Here's the drawing with two shaded views (mm, measured from the low corner). I have some questions. A direction names the side the tool comes from. Give positions to 0.01 mm unless a question says otherwise; leave off trailing zeros. Write each loop counter-clockwise with the first axis right and the second up, starting at its lowest first coordinate (ties: lowest second). Pieces come first, ordered by that corner, then holes. Notation, with made-up numbers: (58.25, -13.5) - (103.25, -13.5) arc R7 cw to (103.25, -3.5) - close; hole circle Ø2 at (19, 15.5). An arc over 180 degrees is marked (long way). Write item = value, one per line.
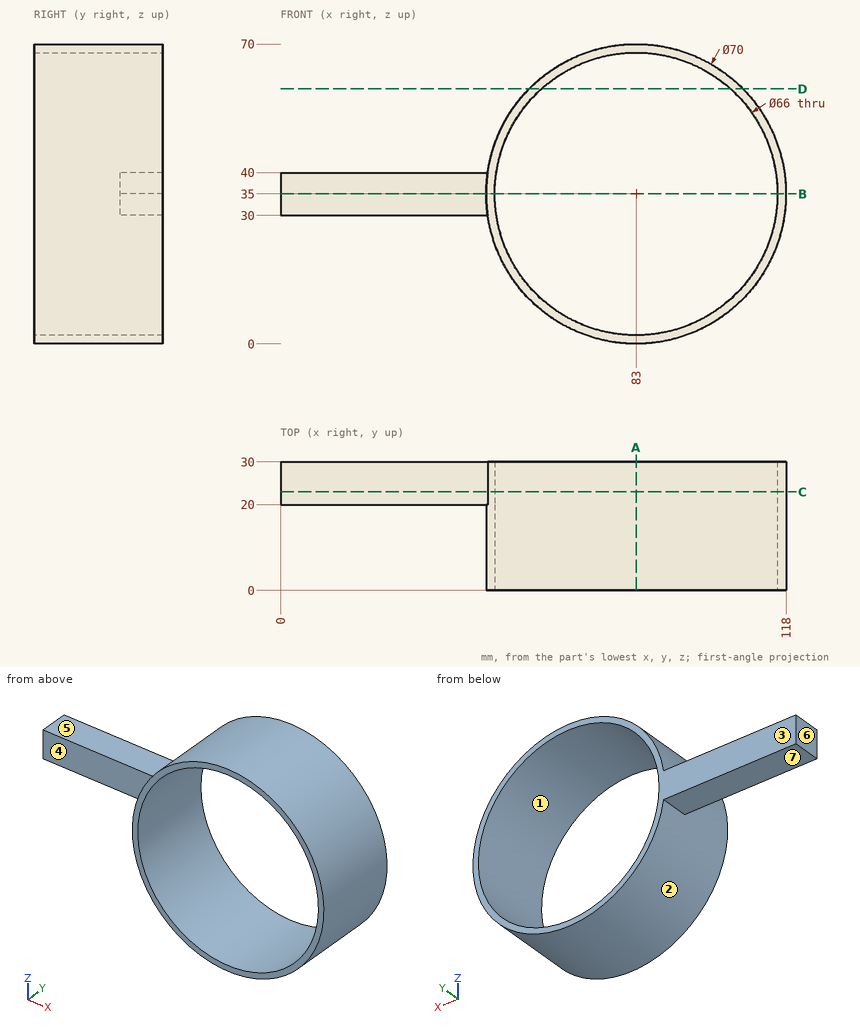
1. I need wall thicknesses on line 1 (Z direction, x = 83, y = 11.75); line 2 (X direction, y = 21.5, z = 35); line 3 (X direction, y = 19.5, z = 35). Which ranges of each line are inside material? Lowest first, please.
Filled sheet:
line_1 = 0 to 2, 68 to 70
line_2 = 0 to 50, 116 to 118
line_3 = 48 to 50, 116 to 118
2. If we section it at B-B, the plane z = 35: Please give me the cut outline in (x, y), and give its area (3 significant figures).
Filled sheet:
outline = (0, 20) - (48, 20) - (48, 0) - (50, 0) - (50, 30) - (0, 30) - close; (116, 0) - (118, 0) - (118, 30) - (116, 30) - close
area = 600 mm2
3. If we section it at A-A, the plane x = 83: Please give me the cut outline in (y, z), and give its area (3 significant figures).
Filled sheet:
outline = (0, 0) - (30, 0) - (30, 2) - (0, 2) - close; (0, 68) - (30, 68) - (30, 70) - (0, 70) - close
area = 120 mm2
4. If we section it at C-C, the plane y = 23: Please give me the cut outline in (x, z).
Filled sheet:
outline = (0, 30) - (48.36, 30) arc R35 ccw (long way) to (48.36, 40) - (0, 40) - close; hole circle Ø66 at (83, 35)
5. If we section it at D-D, the plane z = 59.5: Please give me the cut outline in (x, y) (3 decimals).
Filled sheet:
outline = (58.005, 0) - (60.892, 0) - (60.892, 30) - (58.005, 30) - close; (105.108, 0) - (107.995, 0) - (107.995, 30) - (105.108, 30) - close
6. Thinking about a two-plate mould opening in Z: for the marked faces 1, 2 and 3, which applies, pulls with the +Z half, pulls with the -Z half, needs draft (parallel to the pull), parting line crosses it, or undercut?
Filled sheet:
face_1 = undercut
face_2 = parting line crosses it
face_3 = needs draft
7. For pin 1 (5 mm diameter, centred on x = 15, z = 33.5, fed in from -Y); pin 2 (2 mm diameter, centred on x = 89.5, y = 5, fed in from -Z); pin 3 (3 mm diameter, centred on y = 22, z = 11.5, fed in from +X), each with a flat end and sliding along its axis, tell me the tip position at first contact or that it passes through.
Filled sheet:
pin_1 = 20
pin_2 = 0.43
pin_3 = 110.22
8. Which directions (+Z, -Z, +X, -X, +Y, -Y) give clear straight access to the entire face, cutting with the end or side of a thin tool? Please do the marked faces 4, 5, 6 and 7.
Filled sheet:
face_4 = +Z, -Z, -X, -Y
face_5 = +Z, -X, +Y, -Y
face_6 = +Z, -Z, -X, +Y, -Y
face_7 = -Z, -X, +Y, -Y
